Source: CAD feature listing. Evaluate the final solid. Frame: model axes, mm. Give positions to 0.01 mm unless a question says otherwise; leave off trailing zeros. Loops run counter-clockwise (first coordinate to the right, second up) from the corner with the lowest first, then second, coordinate; pieces in that order, holes last. Notation, with made-up numbers: M 33,69 L 67,69 A25 cw 67,105 Z; hole C -11,53.25 d11. An arc over 180 degrees is marked long. Answer in a Markdown table with one row per item.
```python
from build123d import *

# Parameters (mm, degrees)
SKETCH1_R           = 1.6
SKETCH1_R_2         = 1.15
SKETCH1_R_3         = 4.15
BOSS_EXTRUDE2_DEPTH = 1.7


with BuildPart() as part:
    # Sketch1 → Boss-Extrude2 (new body)
    with BuildSketch(Plane(origin=(0, 0, 0), x_dir=(1, 0, 0), z_dir=(0, 1, 0))):
        with BuildLine():
            Line((1.803573736, -32.521333333), (15.999444435, -22.366666667))
            ThreePointArc((15.999444435, -22.366666667), (19.445436483, -19.445436483), (22.366666667, -15.999444435))
            Line((22.366666667, -15.999444435), (32.521333333, -1.803573736))
            ThreePointArc((32.521333333, -1.803573736), (33.1, 0), (32.521333333, 1.803573736))
            Line((32.521333333, 1.803573736), (22.366666667, 15.999444435))
            ThreePointArc((22.366666667, 15.999444435), (19.445436483, 19.445436483), (15.999444435, 22.366666667))
            Line((15.999444435, 22.366666667), (1.803573736, 32.521333333))
            ThreePointArc((1.803573736, 32.521333333), (0, 33.1), (-1.803573736, 32.521333333))
            Line((-1.803573736, 32.521333333), (-15.999444435, 22.366666667))
            ThreePointArc((-15.999444435, 22.366666667), (-19.445436483, 19.445436483), (-22.366666667, 15.999444435))
            Line((-22.366666667, 15.999444435), (-32.521333333, 1.803573736))
            ThreePointArc((-32.521333333, 1.803573736), (-33.1, 0), (-32.521333333, -1.803573736))
            Line((-32.521333333, -1.803573736), (-22.366666667, -15.999444435))
            ThreePointArc((-22.366666667, -15.999444435), (-19.445436483, -19.445436483), (-15.999444435, -22.366666667))
            Line((-15.999444435, -22.366666667), (-1.803573736, -32.521333333))
            ThreePointArc((-1.803573736, -32.521333333), (0, -33.1), (1.803573736, -32.521333333))
        make_face()
        with Locations(Location((0, -30, 0), (0, 0, 270))):
            Circle(SKETCH1_R, mode=Mode.SUBTRACT)
        with Locations(Location((0, 9, 0), (0, 0, 270))):
            Circle(SKETCH1_R_2, mode=Mode.SUBTRACT)
        with Locations(Location((-7.794228634, -4.5, 0), (0, 0, 270))):
            Circle(SKETCH1_R_2, mode=Mode.SUBTRACT)
        with Locations(Location((7.794228634, -4.5, 0), (0, 0, 270))):
            Circle(SKETCH1_R_2, mode=Mode.SUBTRACT)
        with Locations(Location((0, 0, 0), (0, 0, 270))):
            Circle(SKETCH1_R_3, mode=Mode.SUBTRACT)
        with Locations(Location((30, 0, 0), (0, 0, 270))):
            Circle(SKETCH1_R, mode=Mode.SUBTRACT)
        with Locations(Location((-30, 0, 0), (0, 0, 270))):
            Circle(SKETCH1_R, mode=Mode.SUBTRACT)
        with Locations(Location((0, 30, 0), (0, 0, 270))):
            Circle(SKETCH1_R, mode=Mode.SUBTRACT)
    extrude(amount=BOSS_EXTRUDE2_DEPTH)


solid = part.part
```
Q1. Section query D-D (y = 0.85). Give the number of separate pieces and of enclosed holes in the cut face, plus the area to 3 significant figures.
Values follow:
| item | result |
|---|---|
| separate pieces | 1 |
| enclosed holes | 8 |
| area | 2,560 mm^2 |
Q2. Section query C-C (x = 30). Output: boundary loops of the cut face in (y, z).
Values follow:
| item | result |
|---|---|
| outline | M 0,-5.33 L 1.7,-5.33 L 1.7,-1.6 L 0,-1.6 Z; M 0,1.6 L 1.7,1.6 L 1.7,5.33 L 0,5.33 Z |
Q3. Ray query, probe 1 along X at (y, z) = (0.95, 0); probe 2 along X at (y, z) = (1.2, 4.5); probe 3 along X at (y, z) = (0.45, 30.5). Return the intervals inside material, ascending. Write a range as from..to.
Values follow:
| item | result |
|---|---|
| probe 1 | -33.1..-31.6, -28.4..-4.15, 4.15..28.4, 31.6..33.1 |
| probe 2 | -30.59..-8.94, -6.64..6.64, 8.94..30.59 |
| probe 3 | -4.63..-1.52, 1.52..4.63 |
Q4. Mould query, pull axis X, two halves, no side actions, for faces 1 (the cylindrical face through (19.4, 0.84, 19.49)), 2 (the cylindrical face through (-28.414, 0.838, -0.208)), 3 (the flat face through (0, 1.7, 7)). Classes: +X half, -X half, draft (parallel to the pull), parting line (faces both ways), or undercut.
Values follow:
| item | result |
|---|---|
| face 1 | +X half |
| face 2 | undercut |
| face 3 | draft |
Q5. Section query A-A (x = 0). Output: boundary loops of the cut face in (y, z), plus the area to 3 significant figures.
Values follow:
| item | result |
|---|---|
| outline | M 0,-33.1 L 1.7,-33.1 L 1.7,-31.6 L 0,-31.6 Z; M 0,-28.4 L 1.7,-28.4 L 1.7,-10.15 L 0,-10.15 Z; M 0,-7.85 L 1.7,-7.85 L 1.7,-4.15 L 0,-4.15 Z; M 0,4.15 L 1.7,4.15 L 1.7,28.4 L 0,28.4 Z; M 0,31.6 L 1.7,31.6 L 1.7,33.1 L 0,33.1 Z |
| area | 83.6 mm^2 |
Q6. Section query B-B (z = 0). Output: boundary loops of the cut face in (x, y), plus the area to 4 significant figures.
Values follow:
| item | result |
|---|---|
| outline | M -33.1,0 L -31.6,0 L -31.6,1.7 L -33.1,1.7 Z; M -28.4,0 L -4.15,0 L -4.15,1.7 L -28.4,1.7 Z; M 4.15,0 L 28.4,0 L 28.4,1.7 L 4.15,1.7 Z; M 31.6,0 L 33.1,0 L 33.1,1.7 L 31.6,1.7 Z |
| area | 87.55 mm^2 |
Q7. Contact query for flat-ended pins moving along their axis: pin 1 Ø6.5 at (x, z) = (0, 0) entering from +Y; pin 2 Ø2.5 at (x, z) = (0, -9) entering from +Y. Output: stop coordinate, or through.
Values follow:
| item | result |
|---|---|
| pin 1 | through |
| pin 2 | y = 1.7 |
